from build123d import *

# Parameters (mm, degrees)
SKETCH1_R           = 55
SKETCH1_R_2         = 5
BOSS_EXTRUDE1_DEPTH = 1.5
SKETCH2_R           = 1.5
CUT_EXTRUDE1_DEPTH  = 1.5


with BuildPart() as part:
    # Sketch1 → Boss-Extrude1 (new body)
    with BuildSketch(Plane(origin=(0, 0, 0), x_dir=(1, 0, 0), z_dir=(0, 1, 0))):
        with Locations(Location((0, 0, 0), (0, 0, 270))):
            Circle(SKETCH1_R)
        with Locations(Location((0, 0, 0), (0, 0, 270))):
            Circle(SKETCH1_R_2, mode=Mode.SUBTRACT)
        with BuildLine():
            Line((8, 33.941125497), (8, 12))
            ThreePointArc((8, 12), (9.171572875, 9.171572875), (12, 8))
            Line((12, 8), (33.941125497, 8))
            ThreePointArc((33.941125497, 8), (37.207111821, 9.690598923), (37.712361663, 13.333333333))
            ThreePointArc((37.712361663, 13.333333333), (28.284271247, 28.284271247), (13.333333333, 37.712361663))
            ThreePointArc((13.333333333, 37.712361663), (9.690598923, 37.207111821), (8, 33.941125497))
        make_face(mode=Mode.SUBTRACT)
        with BuildLine():
            Line((-33.941125497, 8), (-12, 8))
            ThreePointArc((-12, 8), (-9.171572875, 9.171572875), (-8, 12))
            Line((-8, 12), (-8, 33.941125497))
            ThreePointArc((-8, 33.941125497), (-9.690598923, 37.207111821), (-13.333333333, 37.712361663))
            ThreePointArc((-13.333333333, 37.712361663), (-28.284271247, 28.284271247), (-37.712361663, 13.333333333))
            ThreePointArc((-37.712361663, 13.333333333), (-37.207111821, 9.690598923), (-33.941125497, 8))
        make_face(mode=Mode.SUBTRACT)
        with BuildLine():
            Line((-33.941125497, -8), (-12, -8))
            ThreePointArc((-12, -8), (-9.171572875, -9.171572875), (-8, -12))
            Line((-8, -12), (-8, -33.941125497))
            ThreePointArc((-8, -33.941125497), (-9.690598923, -37.207111821), (-13.333333333, -37.712361663))
            ThreePointArc((-13.333333333, -37.712361663), (-28.284271247, -28.284271247), (-37.712361663, -13.333333333))
            ThreePointArc((-37.712361663, -13.333333333), (-37.207111821, -9.690598923), (-33.941125497, -8))
        make_face(mode=Mode.SUBTRACT)
        with BuildLine():
            Line((12, -8), (33.941125497, -8))
            ThreePointArc((33.941125497, -8), (37.207111821, -9.690598923), (37.712361663, -13.333333333))
            ThreePointArc((37.712361663, -13.333333333), (28.284271247, -28.284271247), (13.333333333, -37.712361663))
            ThreePointArc((13.333333333, -37.712361663), (9.690598923, -37.207111821), (8, -33.941125497))
            Line((8, -33.941125497), (8, -12))
            ThreePointArc((8, -12), (9.171572875, -9.171572875), (12, -8))
        make_face(mode=Mode.SUBTRACT)
    extrude(amount=-BOSS_EXTRUDE1_DEPTH)

    # Sketch2 → Cut-Extrude1 (cut)
    with BuildSketch(Plane(origin=(0, 0, 0), x_dir=(1, 0, 0), z_dir=(0, 1, 0))):
        with Locations(Location((10, 0, 0), (0, 0, 270))):
            Circle(SKETCH2_R)
        with Locations(Location((7.071067812, -7.071067812, 0), (0, 0, 270))):
            Circle(SKETCH2_R)
        with Locations(Location((0, -10, 0), (0, 0, 270))):
            Circle(SKETCH2_R)
        with Locations(Location((-7.071067812, -7.071067812, 0), (0, 0, 270))):
            Circle(SKETCH2_R)
        with Locations(Location((-10, 0, 0), (0, 0, 270))):
            Circle(SKETCH2_R)
        with Locations(Location((-7.071067812, 7.071067812, 0), (0, 0, 270))):
            Circle(SKETCH2_R)
        with Locations(Location((0, 10, 0), (0, 0, 270))):
            Circle(SKETCH2_R)
        with Locations(Location((7.071067812, 7.071067812, 0), (0, 0, 270))):
            Circle(SKETCH2_R)
        with Locations(Location((-44.316348886, 7.814167995, 0), (0, 0, 270))):
            Circle(SKETCH2_R)
        with Locations(Location((-44.316348886, -7.814167995, 0), (0, 0, 90))):
            Circle(SKETCH2_R)
        with Locations(Location((7.934714132, 45, 0), (0, 0, 270))):
            Circle(SKETCH2_R)
        with Locations(Location((-7.934714132, 45, 0), (0, 0, 90))):
            Circle(SKETCH2_R)
        with Locations(Location((44.316348886, -7.814167995, 0), (0, 0, 270))):
            Circle(SKETCH2_R)
        with Locations(Location((44.316348886, 7.814167995, 0), (0, 0, 90))):
            Circle(SKETCH2_R)
        with Locations(Location((-7.814167995, -44.316348886, 0), (0, 0, 270))):
            Circle(SKETCH2_R)
        with Locations(Location((7.814167995, -44.316348886, 0), (0, 0, 90))):
            Circle(SKETCH2_R)
    extrude(amount=-CUT_EXTRUDE1_DEPTH, mode=Mode.SUBTRACT)


solid = part.part
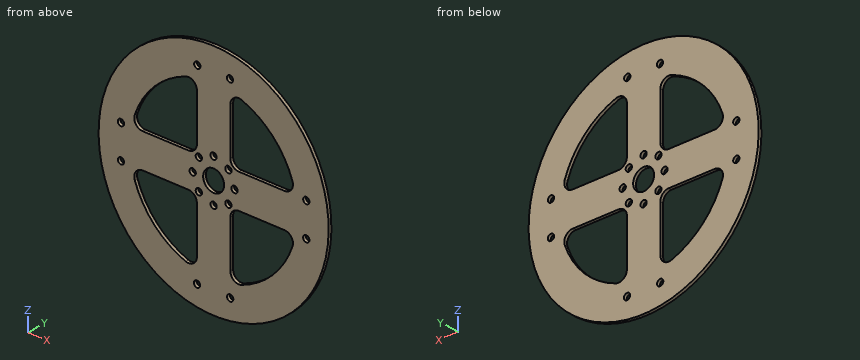
CAD build for the part. Positions are in the model's coordinates, mm. Round coordinates to 2 decimals unless told otherwise and drop trailing zeros. Loops run counter-clockwise (first coordinate to the right, second up) from the corner with the lowest first, then second, coordinate; pieces in that order, holes last. Notation, with made-up numbers: M 61,-12 L 93,-12 A23 ccw 93,0 Z; hole C 63.25,-24 d10. An arc over 180 degrees is marked long. One line per question, with ' | ' between items. Start each with the question number.
Item 1: Pin check, flat tips, straight feed: pin 1 Ø2.5 at (x, z) = (-44.32, 7.81) entering from -Y; pin 2 Ø0.8 at (x, y) = (-26, -0.5) entering from -Z. Stop position of each tip, or through.
Item 2: Cut at D-D, the plane x = -32.5. Write the cut outline in (y, z), plus the area to 3 significant figures.
Item 3: Cut at B-B, the plane x = 0. Write the cut outline in (y, z), plus the area to 3 significant figures.
Item 4: Cut at A-A, the plane z = 0. Write the cut outline in (x, y).
Item 5: Cut at C-C, the plane z = 18.5. Write the cut outline in (x, y).
Item 6: Wall check: line 1 (X direction, y = -0.4, z = 0); line 2 (X direction, y = -1.4, z = -29.5); line 3 (X direction, y = -1.35, z = 17). Give the ranges that are in metal, low to high.
Responses:
1) pin 1: passes through | pin 2: stops at z = -48.68
2) outline: M -1.5,-44.37 L 0,-44.37 L 0,-23.32 L -1.5,-23.32 Z; M -1.5,-8 L 0,-8 L 0,8 L -1.5,8 Z; M -1.5,23.32 L 0,23.32 L 0,44.37 L -1.5,44.37 Z | area: 87.2 mm²
3) outline: M -1.5,-55 L 0,-55 L 0,-11.5 L -1.5,-11.5 Z; M -1.5,-8.5 L 0,-8.5 L 0,-5 L -1.5,-5 Z; M -1.5,5 L 0,5 L 0,8.5 L -1.5,8.5 Z; M -1.5,11.5 L 0,11.5 L 0,55 L -1.5,55 Z | area: 141 mm²
4) outline: M -55,-1.5 L -11.5,-1.5 L -11.5,0 L -55,0 Z; M -8.5,-1.5 L -5,-1.5 L -5,0 L -8.5,0 Z; M 5,-1.5 L 8.5,-1.5 L 8.5,0 L 5,0 Z; M 11.5,-1.5 L 55,-1.5 L 55,0 L 11.5,0 Z
5) outline: M -51.8,-1.5 L -35.46,-1.5 L -35.46,0 L -51.8,0 Z; M -8,-1.5 L 8,-1.5 L 8,0 L -8,0 Z; M 35.46,-1.5 L 51.8,-1.5 L 51.8,0 L 35.46,0 Z
6) line 1: x = -55 to -11.5, -8.5 to -5, 5 to 8.5, 11.5 to 55 | line 2: x = -46.42 to -27.01, -8 to 8, 27.01 to 46.42 | line 3: x = -52.31 to -36.21, -8 to 8, 36.21 to 52.31
